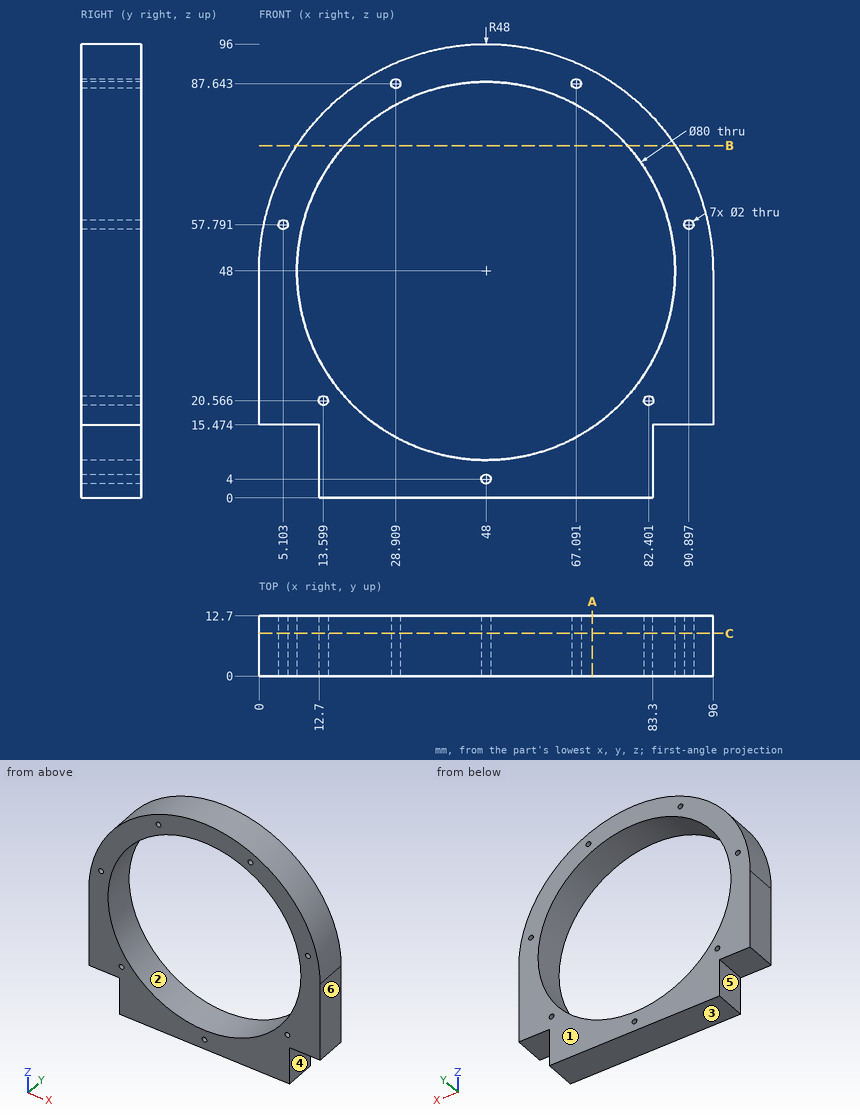
Source: three-view drawing plus pictorial views. Frame: mm from the lowest corner of the part. A direction names the side the tool comes from. Coordinates: 2 decimals unless noted, no trailing zeros. Write each loop counter-clockwise with the first axis right and the second up, starting at its lowest first coordinate (ties: lowest second). Pieces come first, ordered by that corner, then holes. Notation, with made-up numbers: (16.25, 39.25) -> (53.25, 39.25) arc R8 cw to (53.25, 44.25) -> close; hole circle Ø5 at (44, 15). An arc over 180 degrees is marked (long way). Answer as a JSON object with one key per item and string values.
1. Mould query, pull axis Z, two halves, no side actions, for the marked faces 1, 2 and 3. Classes: released by +Z, released by -Z, zero draft, split by the parting line, or undercut.
Result set:
{"face 1": "zero draft", "face 2": "undercut", "face 3": "released by -Z"}
2. Section B-B on z = 74.5. Return the cut outline in (x, y).
Result set:
{"outline": "(7.98, 0) -> (18.04, 0) -> (18.04, 12.7) -> (7.98, 12.7) -> close; (77.96, 0) -> (88.02, 0) -> (88.02, 12.7) -> (77.96, 12.7) -> close"}
3. Material intervals for line 1 (Z direction, x = 13.5, y = 5.75) (1 decimal); line 2 (X direction, y = 7.5, z = 48); line 3 (X direction, y = 2, z = 58) (1 decimal), sorted ascending. Write a range as from..to.
Result set:
{"line 1": "z = 0..19.6, 21.6..27.8, 68.2..81.4", "line 2": "x = 0..8, 88..96", "line 3": "x = 1.1..4.1, 6.1..9.3, 86.7..89.9, 91.9..94.9"}
4. Access query for the marked faces 4, 5 and 6. Directions: +Z, -Z, +X, -X, +Y, -Y. A direction counts if a zero-diameter tool reaches every point of the face in a straight line with its end or side. Return the directions, or none.
Result set:
{"face 4": "-Z, +X, +Y, -Y", "face 5": "-Z, -X, +Y, -Y", "face 6": "+Z, -Z, +X, +Y, -Y"}
5. First-contact query: P1, Ø6.5, axis at x = 91.5, y = 4.5, coming from the -Z side; P2, Ø6.5, axis at y = 5.5, z = 10, coming from the +X side; P3, Ø6, axis at x = 77, y = 10, coming from the +Z side. Flat tips, straight axial feed; report the tip coordinate or a pass-through.
Result set:
{"P1": "stops at z = 15.47", "P2": "stops at x = 83.3", "P3": "stops at z = 88.35"}
6. Section C-C on y = 9. Count the separate pieces of the cut face and the enclosed holes in it.
Result set:
{"separate pieces": "1", "enclosed holes": "8"}
7. Section A-A on x = 70.5. Return the cut outline in (y, z), then the cut area to 3 significant figures.
Result set:
{"outline": "(0, 0) -> (12.7, 0) -> (12.7, 14.93) -> (0, 14.93) -> close; (0, 81.07) -> (12.7, 81.07) -> (12.7, 90.4) -> (0, 90.4) -> close", "area": "308 mm2"}
